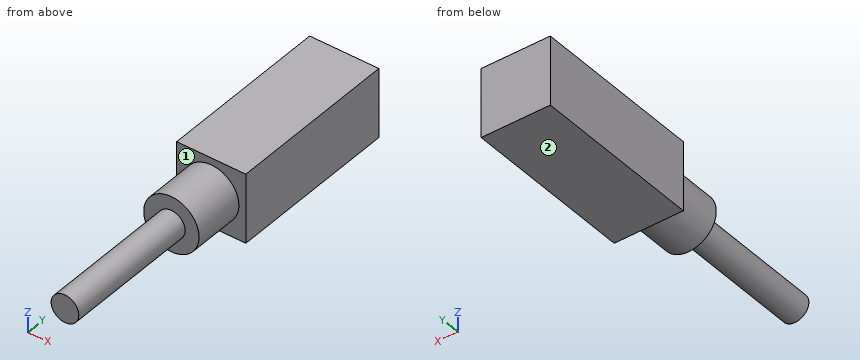
from build123d import *

# Parameters (mm, degrees)
F0_W     = 20
F0_H     = 20
F1_DEPTH = 50
F2_R     = 8
F3_DEPTH = 15
F4_R     = 4
F5_DEPTH = 40


with BuildPart() as f1:
    # F0 (on Front) → F1 (new body)
    with BuildSketch(Plane.XZ):
        with Locations((10, 10)):
            Rectangle(F0_W, F0_H)
    extrude(amount=F1_DEPTH)

    # F2 (on face) → F3 (join)
    with BuildSketch(Plane.XZ.offset(50)):
        with Locations((10, 10)):
            Circle(F2_R)
    extrude(amount=F3_DEPTH)

    # F4 (on face) → F5 (join)
    with BuildSketch(Plane.XZ.offset(65)):
        with Locations((10, 10)):
            Circle(F4_R)
    extrude(amount=F5_DEPTH)


solid = f1.part
Geometry check sheet. Reference: the model listing, model coordinates, mm. Face numbers are marked on the shaded views. A direction names the side the tool comes from. Coordinates: 2 decimals unless noted, no trailing zeros. Order: outer loops, then holes, each group sorted by start corner. A loop starts at its lowest first (then second) coordinate and runs counter-clockwise, first axis right, second up. Notation, with made-up numbers: (-31.75, 39) - (-17.75, 39) arc R23 cw to (-17.75, 53) - close; hole circle Ø6 at (-3.75, -16). An arc over 180 degrees is marked (long way). Answer in a Markdown table with one row per item. Add a question column.
1) Cross-section at D-D, the plane z = 3. Record the cut outline in (x, y).
2) Cross-section at B-B, the plane x = 10. Record the cut outline in (y, z), then the cut area to 3 significant figures.
3) Cross-section at C-C, the plane y = -82. Record the cut outline in (x, z).
4) Material ranges on line 1 along Z through (x, y) = (10.25, -87); line 2 along Y through (x, z) = (13.75, 16.25); line 3 along Y through (x, z) = (15.75, 17.25), recorded low to high. Write a range as [from, to].
5) Cross-section at A-A, the plane z = 10. Record the cut outline in (x, y).
6) Gauge pin test, flat ends, axial feed: P1, Ø6, axis at x = 11, y = -71.5, coming from the +Z side; P2, Ø4, axis at x = 3, y = -76, coming from the +Z side; P3, Ø2, axis at x = 13.5, y = -92, coming from the +Z side; P4, Ø10, axis at y = -64.5, z = 16, coming from the -X side. Record the tip position at first contact, or that the pin passes through.
7) Set-up check for the marked faces 1 and 2: record each of +Z, -Z, +X, -X, +Y, -Y from which the full face is reachable in a straight line by a thin tool's end or side.
Check result:
| question | item | result |
|---|---|---|
| 1 | outline | (0, -50) - (6.13, -50) - (6.13, -65) - (13.87, -65) - (13.87, -50) - (20, -50) - (20, 0) - (0, 0) - close |
| 2 | outline | (-105, 6) - (-65, 6) - (-65, 2) - (-50, 2) - (-50, 0) - (0, 0) - (0, 20) - (-50, 20) - (-50, 18) - (-65, 18) - (-65, 14) - (-105, 14) - close |
| 2 | area | 1,560 mm² |
| 3 | outline | circle Ø8 at (10, 10) |
| 4 | line 1 | z = [6.01, 13.99] |
| 4 | line 2 | y = [-65, 0] |
| 4 | line 3 | y = [-50, 0] |
| 5 | outline | (0, -50) - (2, -50) - (2, -65) - (6, -65) - (6, -105) - (14, -105) - (14, -65) - (18, -65) - (18, -50) - (20, -50) - (20, 0) - (0, 0) - close |
| 6 | P1 | stops at z = 14 |
| 6 | P2 | passes through |
| 6 | P3 | stops at z = 13.12 |
| 6 | P4 | stops at x = 2.06 |
| 7 | face 1 | -Y |
| 7 | face 2 | -Z, +X, -X, +Y, -Y |
